```python
from build123d import *

# Parameters (mm, degrees)
BOSS_EXTRU_1_DEPTH      = 40
ENL_V_MAT_EXTRU_1_REACH = 110.167
ESQUISSE2_W             = 48
ESQUISSE2_H             = 20
ENL_V_MAT_EXTRU_2_REACH = 110.167
ESQUISSE3_R             = 1.25
BOSS_EXTRU_3_DEPTH      = 40


with BuildPart() as part:
    # Esquisse1 → Boss.-Extru.1 (new body)
    with BuildSketch(Plane.XY):
        Polygon((0, 0), (10, 0), (10, 3), (16, 3), (16, 0), (84, 0), (84, 3), (90, 3), (90, 0), (100, 0), (100, 10), (0, 10), align=None)
    extrude(amount=BOSS_EXTRU_1_DEPTH)

    # Esquisse2 → Enlèv. mat.-Extru.1 (cut, up to next)
    with BuildSketch(Plane(origin=(0, 10, 0), x_dir=(1, 0, 0), z_dir=(0, 1, 0)), mode=Mode.PRIVATE) as enl_v_mat_extru_1_sk1:
        with Locations((50, -20)):
            Rectangle(ESQUISSE2_W, ESQUISSE2_H)
    enl_v_mat_extru_1_tool1 = extrude(enl_v_mat_extru_1_sk1.sketch, amount=-ENL_V_MAT_EXTRU_1_REACH, mode=Mode.PRIVATE) & part.part
    add(enl_v_mat_extru_1_tool1.solids().sort_by_distance((50, 10, 20))[0], mode=Mode.SUBTRACT)

    # Esquisse3 → Enlèv. mat.-Extru.2 (cut, up to next)
    with BuildSketch(Plane.XZ, mode=Mode.PRIVATE) as enl_v_mat_extru_2_sk1:
        with Locations(Location((5, 35, 0), (0, 0, 270))):
            Circle(ESQUISSE3_R)
    enl_v_mat_extru_2_tool1 = extrude(enl_v_mat_extru_2_sk1.sketch, amount=-ENL_V_MAT_EXTRU_2_REACH, mode=Mode.PRIVATE) & part.part
    # Esquisse3 → Enlèv. mat.-Extru.2 (cut, up to next)
    with BuildSketch(Plane.XZ, mode=Mode.PRIVATE) as enl_v_mat_extru_2_sk2:
        with Locations(Location((5, 5, 0), (0, 0, 270))):
            Circle(ESQUISSE3_R)
    enl_v_mat_extru_2_tool2 = extrude(enl_v_mat_extru_2_sk2.sketch, amount=-ENL_V_MAT_EXTRU_2_REACH, mode=Mode.PRIVATE) & part.part
    # Esquisse3 → Enlèv. mat.-Extru.2 (cut, up to next)
    with BuildSketch(Plane.XZ, mode=Mode.PRIVATE) as enl_v_mat_extru_2_sk3:
        with Locations(Location((95, 35, 0), (0, 0, 270))):
            Circle(ESQUISSE3_R)
    enl_v_mat_extru_2_tool3 = extrude(enl_v_mat_extru_2_sk3.sketch, amount=-ENL_V_MAT_EXTRU_2_REACH, mode=Mode.PRIVATE) & part.part
    # Esquisse3 → Enlèv. mat.-Extru.2 (cut, up to next)
    with BuildSketch(Plane.XZ, mode=Mode.PRIVATE) as enl_v_mat_extru_2_sk4:
        with Locations(Location((95, 5, 0), (0, 0, 270))):
            Circle(ESQUISSE3_R)
    enl_v_mat_extru_2_tool4 = extrude(enl_v_mat_extru_2_sk4.sketch, amount=-ENL_V_MAT_EXTRU_2_REACH, mode=Mode.PRIVATE) & part.part
    add(enl_v_mat_extru_2_tool1.solids().sort_by_distance((5, 0, 35))[0], mode=Mode.SUBTRACT)
    add(enl_v_mat_extru_2_tool2.solids().sort_by_distance((5, 0, 5))[0], mode=Mode.SUBTRACT)
    add(enl_v_mat_extru_2_tool3.solids().sort_by_distance((95, 0, 35))[0], mode=Mode.SUBTRACT)
    add(enl_v_mat_extru_2_tool4.solids().sort_by_distance((95, 0, 5))[0], mode=Mode.SUBTRACT)

    # Esquisse4 → Boss.-Extru.3 (add)
    with BuildSketch(Plane(origin=(0, 0, 0), x_dir=(-1, 0, 0), z_dir=(0, 0, -1))):
        Polygon((-100, 10), (-112, 10), (-110, 33.2), (-106, 33.7), (-106, 36.2), (-115, 36.2), (-115, 7), (-108, 0), (-100, 0), align=None)
    extrude(amount=-BOSS_EXTRU_3_DEPTH)


solid = part.part
```
Source: CAD feature listing. Evaluate the final solid. Frame: model axes, mm. A direction names the side the tool comes from. Give positions to 0.01 mm unless a question says otherwise; leave off trailing zeros. Loops run counter-clockwise (first coordinate to the right, second up) from the corner with the lowest first, then second, coordinate; pieces in that order, holes last. Notation, with made-up numbers: M 40.5,-12 L 96.5,-12 A16 cw 96.5,6 Z; hole C 34,14 d1. An arc over 180 degrees is marked long. Put each result on its own line as item: value.
Q1. Section C-C (x = 95). Return the cut outline in (y, z).
Response values:
outline: M 0,0 L 10,0 L 10,3.75 L 0,3.75 Z; M 0,6.25 L 10,6.25 L 10,33.75 L 0,33.75 Z; M 0,36.25 L 10,36.25 L 10,40 L 0,40 Z
Q2. Section A-A (x = 69.5). Return the cut outline in (y, z), and give its area (3 significant figures).
Response values:
outline: M 0,0 L 10,0 L 10,10 L 0,10 Z; M 0,30 L 10,30 L 10,40 L 0,40 Z
area: 200 mm²
Q3. Section D-D (z = 5). Return the cut outline in (x, y), and give its area (3 significant figures).
Response values:
outline: M 0,0 L 3.75,0 L 3.75,10 L 0,10 Z; M 6.25,0 L 10,0 L 10,3 L 16,3 L 16,0 L 84,0 L 84,3 L 90,3 L 90,0 L 93.75,0 L 93.75,10 L 6.25,10 Z; M 96.25,0 L 108,0 L 115,7 L 115,36.2 L 106,36.2 L 106,33.7 L 110,33.2 L 112,10 L 96.25,10 Z
area: 1,160 mm²
Q4. Reachability of faces 4 (the flat face through (115, 22, 20)), 5 (the flat face through (26, 5, 20)), 6 (the flat face through (84, 1, 20)) from +Z, -Z, +X, -X, +Y, -Y: full face, straight path, thin tool, end or side. Return the list, or none.
Response values:
face 4: +Z, -Z, +X, +Y, -Y
face 5: +Y, -Y
face 6: +Z, -Z, -Y
Q5. Mould query, pull axis X, two halves, no side actions, for faces 1 (the flat face through (106, 35, 20)), 2 (the flat face through (5, 0, 20)), 3 (the flat face through (13, 3, 20)). Classes: released by +X, released by -X, zero draft, split by the parting line, or undercut.
Response values:
face 1: released by -X
face 2: zero draft
face 3: undercut
Q6. Section B-B (z = 17.5). Return the cut outline in (x, y).
Response values:
outline: M 0,0 L 10,0 L 10,3 L 16,3 L 16,0 L 26,0 L 26,10 L 0,10 Z; M 74,0 L 84,0 L 84,3 L 90,3 L 90,0 L 108,0 L 115,7 L 115,36.2 L 106,36.2 L 106,33.7 L 110,33.2 L 112,10 L 74,10 Z
Q7. Pin query (flat end, axial travel): P1, Ø3, axis at x = 95, z = 5, coming from the +Y side; P2, Ø3.5, axis at y = 1, z = 18.5, coming from the -X side; P3, Ø0.9, axis at y = 1, z = 30, coming from the +X side; P4, Ø1.5, axis at x = 5, z = 35, coming from the +Y side. Return the tip coordinate at first contact, or that it passes through.
Response values:
P1: stops at y = 10
P2: stops at x = 0
P3: stops at x = 109.45
P4: passes through
Q8. Line query: probe 1 along Z at (x, y) = (95, 2.25); probe 2 along Z at (x, y) = (42, 7.5); probe 3 along Y at (x, z) = (70.5, 2.5). Output: solid intervals per line, ascending. Write a range as [from, to].
Response values:
probe 1: z = [0, 3.75], [6.25, 33.75], [36.25, 40]
probe 2: z = [0, 10], [30, 40]
probe 3: y = [0, 10]
